```python
from build123d import *

# Parameters (mm, degrees)
FILLET1_R                = 2
SKETCH5_R                = 8.5
SKETCH5_R_2              = 7
BOSS_EXTRUDE1_DEPTH      = 0.1
BOSS_EXTRUDE2_DEPTH      = 0.5
BOSS_EXTRUDE2_DEPTH_BACK = 0.5
SKETCH6_R                = 2
SKETCH6_R_2              = 1.5
CUT_EXTRUDE1_DEPTH       = 24.885141976
CUT_EXTRUDE1_DEPTH_BACK  = 24.885141976
SKETCH7_R                = 3.75


with BuildPart() as part:
    # Sketch4 → Revolve1 (revolve)
    with BuildSketch(Plane(origin=(0, 0, 0), x_dir=(0, 0, -1), z_dir=(1, 0, 0))):
        Polygon((0, 0), (-3.75, 0), (-4.25, -0.5), (-4.75, 0), (-8.5, 0), (-8.5, -4), (0, -4), align=None)
    revolve(axis=Axis((0, 1.890471386, 0), (0, -1, 0)))

    # Fillet1
    fillet1_edges = [part.edges().sort_by_distance(p)[0] for p in [
        (0, 0, -8.5),
    ]]
    fillet(fillet1_edges, radius=FILLET1_R)



with BuildPart() as body_2:
    # Sketch5 → Boss-Extrude1 (new body)
    with BuildSketch(Plane.XZ.offset(4)):
        with Locations(Location((0, 0, 0), (0, 0, 90))):
            Circle(SKETCH5_R)
        with Locations(Location((0, 0, 0), (0, 0, 270))):
            Circle(SKETCH5_R_2, mode=Mode.SUBTRACT)
    extrude(amount=BOSS_EXTRUDE1_DEPTH)


with BuildPart() as part_1:
    add(part.part)

    add(body_2.part)  # Boss-Extrude2 merges body 2
    # Sketch6 → Boss-Extrude2 (add, two sides: drawn at the far end of the back side and taken through both)
    # profile 1 of 2: a face of its own
    with BuildSketch(Plane(origin=(0, 0, 0), x_dir=(0, 0, -1), z_dir=(1, 0, 0)).offset(-BOSS_EXTRUDE2_DEPTH_BACK)):
        with BuildLine():
            Line((16.132863069, 0.320027848), (0, 0))
            Line((0, 0), (0, -0.907670556))
            Line((0, -0.907670556), (7.174444166, -0.907670556))
            Line((7.174444166, -0.907670556), (8.5, -4))
            Line((8.5, -4), (16.12184584, -1.999779955))
            Line((16.12184584, -1.999779955), (17.746442499, -4.961787965))
            ThreePointArc((17.746442499, -4.961787965), (17.953109522, -2.732273748), (20.098589091, -2.09167846))
            ThreePointArc((20.098589091, -2.09167846), (17.968839585, -1.127360353), (16.132863069, 0.320027848))
        make_face()
    # profile 2 of 2: a face of its own
    with BuildSketch(Plane(origin=(0, 0, 0), x_dir=(0, 0, -1), z_dir=(1, 0, 0)).offset(-BOSS_EXTRUDE2_DEPTH_BACK)):
        with Locations((19.5, -4)):
            Circle(SKETCH6_R)
        with Locations((19.5, -4)):
            Circle(SKETCH6_R_2, mode=Mode.SUBTRACT)
    extrude(amount=BOSS_EXTRUDE2_DEPTH + BOSS_EXTRUDE2_DEPTH_BACK)

    # Sketch7 → Cut-Extrude1 (cut, two sides: drawn at the far end of the back side and taken through both)
    with BuildSketch(Plane(origin=(0, 0, 0), x_dir=(1, 0, 0), z_dir=(0, 1, 0)).offset(-CUT_EXTRUDE1_DEPTH_BACK)):
        with Locations(Location((0, 0, 0), (0, 0, 97.662255661))):
            Circle(SKETCH7_R)
    extrude(amount=CUT_EXTRUDE1_DEPTH + CUT_EXTRUDE1_DEPTH_BACK, mode=Mode.SUBTRACT)


solid = part_1.part
```
Geometry check sheet. Reference: the model listing, model coordinates, mm. A direction names the side the tool comes from. Round coordinates to 2 decimals unless told otherwise and drop trailing zeros. Order: outer loops, then holes, each group sorted by start corner. A loop starts at its lowest first (then second) coordinate and runs counter-clockwise, first axis right, second up. Notation, with made-up numbers: (6, 39) - (20, 39) arc R18 ccw to (20, 59) - close; hole circle Ø4 at (21.5, -20). An arc over 180 degrees is marked (long way). Use a Markdown table: item, result. Add a question column.
1) Section check B-B (y = -3). Record the cut outline in (x, z).
2) Section check A-A (z = 0). Record the cut outline in (x, y), then the cut area to 3 significant figures.
3) Thickness scan on line 1 along X through (y, z) = (-3.1, 0); line 2 along Z through (x, y) = (-1.5, -2.75); line 3 along X through (y, z) = (-2.5, -11.5). Record the ranges inside material, lowest first.
4) Section check D-D (z = -13). Record the cut outline in (x, y).
5) Mould release check, pull along Z, two halves, no side actions. Record for faces 4 (the flat face through (-7, -4.1, 2)), 5 (the flat face through (-0.007, -3.46, -16.923)), 6 (the cylindrical face through (-0.007, -1.144, -17.997)): released by +Z, released by -Z, zero draft, split by the parting line, or undercut.
6) Gauge pin test, flat ends, axial feed: P1, Ø1.9, axis at y = -4, z = -11, coming from the +X side; P2, Ø1, axis at x = 4.5, z = -5.5, coming from the -Y side; P3, Ø1, axis at x = 4, y = -1, coming from the -Z side. Record the tip position at first contact, or that the pin passes through.
7) Section check C-C (z = -19). Record the cut outline in (x, y).
8) Set-up check for faces 1 (the cylindrical face through (0, -4, -18)), 2 (the flat face through (3, -4, 3)), 3 (the flat face through (-0.007, -3.014, -12.258)): record each of +Z, -Z, +X, -X, +Y, -Y from which the full face is reachable in a straight line by a thin tool's end or side.
Established:
| question | item | result |
|---|---|---|
| 1 | outline | (-0.5, -21.23) - (0.5, -21.23) - (0.5, -20.62) - (-0.5, -20.62) - close; (-0.5, -18.38) - (0.5, -18.38) - (0.5, -16.67) - (-0.5, -16.67) - close; (-0.5, -12.31) - (0.5, -12.31) - (0.5, -8.49) arc R8.5 ccw (long way) to (-0.5, -8.49) - close; hole circle Ø7.5 at (0, 0) |
| 2 | outline | (-8.5, -4.1) - (-7, -4.1) - (-7, -4) - (-3.75, -4) - (-3.75, 0) - (-4.25, -0.5) - (-4.75, 0) - (-6.5, 0) arc R2 ccw to (-8.5, -2) - close; (3.75, -4) - (7, -4) - (7, -4.1) - (8.5, -4.1) - (8.5, -2) arc R2 ccw to (6.5, 0) - (4.75, 0) - (4.25, -0.5) - (3.75, 0) - close |
| 2 | area | 36.1 mm2 |
| 3 | line 1 | -8.5 to -3.75, 3.75 to 8.5 |
| 3 | line 2 | -8.37 to -3.44, 3.44 to 8.37 |
| 3 | line 3 | -0.5 to 0.5 |
| 4 | outline | (-0.5, -2.82) - (0.5, -2.82) - (0.5, 0.26) - (-0.5, 0.26) - close |
| 5 | face 4 | zero draft |
| 5 | face 5 | undercut |
| 5 | face 6 | released by -Z |
| 6 | P1 | x = 0.5 |
| 6 | P2 | y = -4.1 |
| 6 | P3 | z = -7.56 |
| 7 | outline | (-0.5, -5.94) - (0.5, -5.94) - (0.5, -5.41) - (-0.5, -5.41) - close; (-0.5, -2.59) - (0.5, -2.59) - (0.5, -1.67) - (-0.5, -1.67) - close |
| 8 | face 1 | +X, -X |
| 8 | face 2 | -Y |
| 8 | face 3 | +X, -X, -Y |
